Read the model definition and answer for the solid it produces. Units are mm, in the model's axes. A direction names the side the tool comes from. Give positions to 0.01 mm unless a question says otherwise; leave off trailing zeros. Order: outer loops, then holes, each group sorted by start corner. A loop starts at its lowest first (then second) coordinate and runs counter-clockwise, first axis right, second up. Notation, with made-up numbers: (43.25, 35) - (101.25, 35) arc R6 cw to (101.25, 40) - close; hole circle Ø10 at (4, -23). An arc over 180 degrees is marked (long way). Return JSON: item names as keys, results as strings.
```python
from build123d import *

# Parameters (mm, degrees)
SKETCH_1_W      = 55
SKETCH_1_H      = 75
SKETCH_1_R      = 1.75
EXTRUDE_1_DEPTH = 2
SKETCH_2_W      = 55
SKETCH_2_H      = 75
SKETCH_2_W_2    = 53
SKETCH_2_H_2    = 73
EXTRUDE_2_DEPTH = 10


with BuildPart() as part:
    # Эскиз1 → Бобышка-Вытянуть1 (new body)
    with BuildSketch(Plane.XY):
        with Locations((27.5, 37.5)):
            Rectangle(SKETCH_1_W, SKETCH_1_H)
        with Locations((5, 70)):
            Circle(SKETCH_1_R, mode=Mode.SUBTRACT)
        with Locations((50, 70)):
            Circle(SKETCH_1_R, mode=Mode.SUBTRACT)
        with Locations((5, 5)):
            Circle(SKETCH_1_R, mode=Mode.SUBTRACT)
        with Locations((50, 5)):
            Circle(SKETCH_1_R, mode=Mode.SUBTRACT)
    extrude(amount=EXTRUDE_1_DEPTH)

    # Эскиз2 → Бобышка-Вытянуть2 (add)
    with BuildSketch(Plane.XY.offset(2)):
        with Locations((27.5, 37.5)):
            Rectangle(SKETCH_2_W, SKETCH_2_H)
        with Locations((27.5, 37.5)):
            Rectangle(SKETCH_2_W_2, SKETCH_2_H_2, mode=Mode.SUBTRACT)
    extrude(amount=EXTRUDE_2_DEPTH)


solid = part.part
```
Q1. A cutting plane is placed at B-B (y = 5). Write down the section's boundary in (x, z).
Values:
{"outline": "(0, 0) - (3.25, 0) - (3.25, 2) - (1, 2) - (1, 12) - (0, 12) - close; (6.75, 0) - (48.25, 0) - (48.25, 2) - (6.75, 2) - close; (51.75, 0) - (55, 0) - (55, 12) - (54, 12) - (54, 2) - (51.75, 2) - close"}
Q2. A cutting plane is placed at A-A (z = 6.75). Write down the section's boundary in (x, y), and give its area (3 significant figures).
Values:
{"outline": "(0, 0) - (55, 0) - (55, 75) - (0, 75) - close; hole (1, 1) - (54, 1) - (54, 74) - (1, 74) - close", "area": "256 mm²"}
Q3. Determine the mould class of faces 3 (the cylindrical face through (51.617, 4.33, 0.986)), 4 (the flat face through (55, 37, 6)), 5 (the flat face through (27, 38, 0)) for opening direction X: released by +X, released by -X, zero draft, split by the parting line, or undercut.
Values:
{"face 3": "undercut", "face 4": "released by +X", "face 5": "zero draft"}
Q4. A cutting plane is placed at C-C (x = 5). Write down the section's boundary in (y, z).
Values:
{"outline": "(0, 0) - (3.25, 0) - (3.25, 2) - (1, 2) - (1, 12) - (0, 12) - close; (6.75, 0) - (68.25, 0) - (68.25, 2) - (6.75, 2) - close; (71.75, 0) - (75, 0) - (75, 12) - (74, 12) - (74, 2) - (71.75, 2) - close"}
Q5. Given pin 1 (3 mm diameter, centred on x = 50, y = 5, fed in from +Z); pin 2 (12 mm diameter, centred on x = 34, y = 9, fed in from +Z), each flat-ended and moving along its own axis, determine where each tip first touches the part or whether it passes through.
Values:
{"pin 1": "passes through", "pin 2": "stops at z = 2"}
Q6. A cutting plane is placed at D-D (x = 26.5). Write down the section's boundary in (y, z).
Values:
{"outline": "(0, 0) - (75, 0) - (75, 12) - (74, 12) - (74, 2) - (1, 2) - (1, 12) - (0, 12) - close"}
Q7. For faces 1 (the flat face through (27, 74, 7)), 2 (the cylindrical face through (4.62, 68.29, 0.99)), determine the directions among +Z, -Z, +X, -X, +Y, -Y from which every point of the face is accessible in a straight line to the end or side of a thin tool.
Values:
{"face 1": "+Z", "face 2": "+Z, -Z"}
Q8. Consider L1, parallel to Y at x = 50, z = 0.8; L2, parallel to X at y = 70, z = 1.05; L3, parallel to X at y = 33.5, z = 9. Determine where each line is inside the solid, lowest interval first.
Values:
{"L1": "y = 0 to 3.25, 6.75 to 68.25, 71.75 to 75", "L2": "x = 0 to 3.25, 6.75 to 48.25, 51.75 to 55", "L3": "x = 0 to 1, 54 to 55"}
